Read the model definition and answer for the solid it produces. Units are mm, in the model's axes. A direction names the side the tool comes from. Coordinates: 2 decimals unless noted, no trailing zeros. Write each loop counter-clockwise with the first axis right and the second up, starting at its lowest first coordinate (ties: lowest second). Pieces come first, ordered by that corner, then holes. Notation, with made-up numbers: (79.5, 7.25) -> (127.5, 7.25) arc R26 ccw to (127.5, 22.25) -> close; hole circle Ø4 at (28.25, 77). An arc over 180 degrees is marked (long way). Answer in a Markdown table with one row per item. Add a question column.
Item 1: Straight lines are drawn through the part: line 1 (X direction, y = -1.95, z = 15.5); line 2 (Z direction, x = 0, y = -27.85); line 3 (Y direction, x = 14.5, z = -14). For each, find the intervals that lie inside material, in ascending order. Write a range as from..to.
Item 2: Section C-C on z = -5.5 is taken. Write down the section's boundary in (x, y).
Item 3: Section A-A on x = 7 is taken. Write down the section's boundary in (y, z).
Item 4: Section D-D on y = -41 is taken. Write down the section's boundary in (x, z).
Item 5: Section B-B on y = -12 is taken. Write down the section's boundary in (x, z).
Item 6: For a pull along Z with two mould halves and no side action, classify faces 4 (the face through (0, -2, 21)), 5 (the face through (13.926, -2.535, 15.004)), 6 (the face through (9, 0, -9)) as +Z half, -Z half, draft (parallel to the pull), parting line (faces both ways), or undercut.
Item 7: Given pin 1 Ø5.5 at (x, z) = (9.9, -9.9) entering from +Y; pin 2 Ø5.5 at (x, z) = (-15.5, 15.5) entering from -Y; pin 3 Ø0.6 at (x, z) = (0.5, 2) entering from -Y; pin 4 Ø7.5 at (x, z) = (0, 5) entering from +Y, each flat-ended and moving along its own axis, determine where each tip first touches the part or whether it passes through.
Item 8: Which of the six approach directions +Z, -Z, +X, -X, +Y, -Y give full straight-line access (tool end or side, diameter ignored) to faces 1 (the face through (-0.54, -39.61, -2.44)), 2 (the face through (11.923, -2.465, 3.755)), 3 (the face through (21, -2, 0))?
```python
from build123d import *

# Parameters (mm, degrees)
F0_W     = 42
F0_H     = 42
F0_R     = 12.5
F1_DEPTH = 5
F2_R     = 18
F2_R_2   = 12.5
F3_DEPTH = 25
F4_R     = 2.5
F5_DEPTH = 20
F7_DEPTH = 15
F8_D     = 3.3
F9_D     = 3.3
F9_DEPTH = 6
F9_TIP   = 0.9914200214
F10_SIZE = 5
F11_SIZE = 0.5


with BuildPart() as f1:
    # F0 (on Front) → F1 (new body)
    with BuildSketch(Plane.XZ):
        Rectangle(F0_W, F0_H)
        Circle(F0_R, mode=Mode.SUBTRACT)
    extrude(amount=F1_DEPTH)

    # F2 (on face) → F3 (join)
    with BuildSketch(Plane.XZ.offset(5)):
        Circle(F2_R)
        Circle(F2_R_2, mode=Mode.SUBTRACT)
        Circle(F2_R_2)
    extrude(amount=F3_DEPTH)

    # F4 (on face) → F5 (join)
    with BuildSketch(Plane.XZ.offset(30)):
        Circle(F4_R)
    extrude(amount=F5_DEPTH)

    # F6 (on face) → F7 (cut)
    with BuildSketch(Plane.XZ.offset(50)):
        with BuildLine():
            Line((-2, 1.5), (2, 1.5))
            ThreePointArc((2, 1.5), (0, 2.5), (-2, 1.5))
        make_face()
    extrude(amount=-F7_DEPTH, mode=Mode.SUBTRACT)

    # F8 (through all)
    with Locations(Plane(origin=(0, 0, 0), x_dir=(1, 0, 0), z_dir=(0, 1, 0))):
        with Locations((-15.5, -15.5), (15.5, -15.5), (-15.5, 15.5), (15.5, 15.5)):
            Hole(F8_D / 2)

    # F9
    with Locations(Plane.XZ.offset(30)):
        with Locations((0, 14), (-14, 0), (0, -14), (14, 0), (-9.8994949366, 9.8994949366), (-9.8994949366, -9.8994949366), (9.8994949366, -9.8994949366), (9.8994949366, 9.8994949366)):
            Hole(F9_D / 2, depth=F9_DEPTH)
            with Locations((0, 0, -(F9_DEPTH + F9_TIP / 2))):  # 118° drill point
                Cone(0, F9_D / 2, F9_TIP, mode=Mode.SUBTRACT)

    # F10
    f10_edges = [f1.edges().sort_by_distance(p)[0] for p in [
        (-21, -2.5, 21),
        (21, -2.5, 21),
        (-21, -2.5, -21),
        (21, -2.5, -21),
    ]]
    chamfer(f10_edges, length=F10_SIZE)

    # F11
    f11_edges = [f1.edges().sort_by_distance(p)[0] for p in [
        (-0.790569, -50, -2.371708),
        (0, -35, 2.5),
    ]]
    chamfer(f11_edges, length=F11_SIZE)


solid = f1.part
```
Results below:
| question | item | result |
|---|---|---|
| 1 | line 1 | x = -21..-17.15, -13.85..13.85, 17.15..21 |
| 1 | line 2 | z = -18..-15.65, -12.35..12.35, 15.65..18 |
| 1 | line 3 | y = -5..0 |
| 2 | outline | (-21, -5) -> (-17.14, -5) -> (-17.14, -30) -> (17.14, -30) -> (17.14, -5) -> (21, -5) -> (21, 0) -> (11.22, 0) -> (11.22, -5) -> (-11.22, -5) -> (-11.22, 0) -> (-21, 0) -> close |
| 3 | outline | (-30, -16.58) -> (-5, -16.58) -> (-5, -21) -> (0, -21) -> (0, -10.36) -> (-5, -10.36) -> (-5, 10.36) -> (0, 10.36) -> (0, 21) -> (-5, 21) -> (-5, 16.58) -> (-30, 16.58) -> close |
| 4 | outline | (-2, 1.5) arc R2.5 ccw (long way) to (2, 1.5) -> close |
| 5 | outline | circle Ø36 at (0, 0) |
| 6 | face 4 | +Z half |
| 6 | face 5 | undercut |
| 6 | face 6 | draft |
| 7 | pin 1 | stops at y = 0 |
| 7 | pin 2 | stops at y = -5 |
| 7 | pin 3 | stops at y = -35 |
| 7 | pin 4 | stops at y = -5 |
| 8 | face 1 | -Y |
| 8 | face 2 | +Y |
| 8 | face 3 | +Z, -Z, +X, +Y, -Y |
